from build123d import *

# Parameters (mm, degrees)
SALIENTE_EXTRUIR1_DEPTH = 30
CORTAR_EXTRUIR1_DEPTH   = 5
CROQUIS3_W              = 30.2
CROQUIS3_H              = 25.2
CORTAR_EXTRUIR2_DEPTH   = 2
CROQUIS4_R              = 1.1
CORTAR_EXTRUIR3_DEPTH   = 5
CROQUIS5_W              = 25.2
CROQUIS5_H              = 25.2
CORTAR_EXTRUIR4_DEPTH   = 2
REDONDEO2_R             = 8
REDONDEO3_R             = 2.7
CROQUIS6_W              = 8
CROQUIS6_H              = 14
SALIENTE_EXTRUIR2_DEPTH = 5
REDONDEO4_R             = 3
SALIENTE_EXTRUIR4_START = -2.4
SALIENTE_EXTRUIR4_DEPTH = 2.4
SALIENTE_EXTRUIR5_START = -30
SALIENTE_EXTRUIR5_DEPTH = 2.4
REDONDEO5_R             = 10
SALIENTE_EXTRUIR6_START = -5
SALIENTE_EXTRUIR6_DEPTH = 5
CORTAR_EXTRUIR6_START   = -2.4
CROQUIS14_R             = 1
CORTAR_EXTRUIR6_DEPTH   = 30
CROQUIS18_W             = 3
CROQUIS18_H             = 7.151114147
SALIENTE_EXTRUIR7_DEPTH = 5
CORTAR_EXTRUIR7_START   = -3
CORTAR_EXTRUIR7_DEPTH   = 3
CROQUIS22_R             = 1
CORTAR_EXTRUIR8_DEPTH   = 5
REDONDEO8_R             = 2
REDONDEO6_R             = 3


with BuildPart() as part:
    # Croquis1 → Saliente-Extruir1 (new body)
    with BuildSketch(Plane.XY):
        with BuildLine():
            Line((0, 0), (0, 5))
            Line((0, 5), (-40, 5))
            ThreePointArc((-40, 5), (-58.443639467, -0.437358826), (-71, -15))
            Line((-71, -15), (-71, -55))
            Line((-71, -55), (-66, -55))
            Line((-66, -55), (-66, -16.078431373))
            ThreePointArc((-66, -16.078431373), (-55.744135615, -4.621589797), (-41.078431373, 0))
            Line((-41.078431373, 0), (0, 0))
        make_face()
    extrude(amount=SALIENTE_EXTRUIR1_DEPTH)

    # Croquis2 → Cortar-Extruir1 (cut)
    with BuildSketch(Plane(origin=(0, 5, 0), x_dir=(1, 0, 0), z_dir=(0, 1, 0))):
        with BuildLine():
            Line((-18.4, -7.18), (-8.4, -7.18))
            ThreePointArc((-8.4, -7.18), (-7.3, -8.28), (-8.4, -9.38))
            Line((-8.4, -9.38), (-28.4, -9.38))
            ThreePointArc((-28.4, -9.38), (-29.5, -8.28), (-28.4, -7.18))
            Line((-28.4, -7.18), (-18.4, -7.18))
        make_face()
        with BuildLine():
            Line((-8.4, -20.62), (-28.4, -20.62))
            ThreePointArc((-28.4, -20.62), (-29.5, -21.72), (-28.4, -22.82))
            Line((-28.4, -22.82), (-18.4, -22.82))
            Line((-18.4, -22.82), (-8.4, -22.82))
            ThreePointArc((-8.4, -22.82), (-7.3, -21.72), (-8.4, -20.62))
        make_face()
    extrude(amount=-CORTAR_EXTRUIR1_DEPTH, mode=Mode.SUBTRACT)

    # Croquis3 → Cortar-Extruir2 (cut)
    with BuildSketch(Plane.XZ):
        with Locations((-18.4, 15)):
            Rectangle(CROQUIS3_W, CROQUIS3_H)
    extrude(amount=-CORTAR_EXTRUIR2_DEPTH, mode=Mode.SUBTRACT)

    # Croquis4 → Cortar-Extruir3 (cut)
    with BuildSketch(Plane.ZY.offset(71)):
        with Locations((22.071067812, -29.528932188)):
            Circle(CROQUIS4_R)
        with Locations((22.071067812, -43.671067812)):
            Circle(CROQUIS4_R)
        with Locations((7.928932188, -43.671067812)):
            Circle(CROQUIS4_R)
        with Locations((7.928932188, -29.528932188)):
            Circle(CROQUIS4_R)
    extrude(amount=-CORTAR_EXTRUIR3_DEPTH, mode=Mode.SUBTRACT)

    # Croquis5 → Cortar-Extruir4 (cut)
    with BuildSketch(Plane.ZY.offset(71)):
        with Locations((15, -36.6)):
            Rectangle(CROQUIS5_W, CROQUIS5_H)
    extrude(amount=-CORTAR_EXTRUIR4_DEPTH, mode=Mode.SUBTRACT)

    # Redondeo2
    redondeo2_edges = [part.edges().sort_by_distance(p)[0] for p in [
        (0, 2.5, 0),
        (-71, -15, 15),
        (-68.5, -55, 30),
        (0, 2.5, 30),
        (-68.5, -55, 0),
    ]]
    fillet(redondeo2_edges, radius=REDONDEO2_R)

    # Redondeo3
    redondeo3_edges = [part.edges().sort_by_distance(p)[0] for p in [
        (-70, -24, 27.6),
        (-70, -49.2, 27.6),
        (-70, -49.2, 2.4),
        (-70, -24, 2.4),
        (-3.3, 1, 27.6),
        (-3.3, 1, 2.4),
        (-33.5, 1, 2.4),
        (-33.5, 1, 27.6),
    ]]
    fillet(redondeo3_edges, radius=REDONDEO3_R)

    # Croquis6 → Saliente-Extruir2 (add)
    with BuildSketch(Plane.XZ):
        with Locations((4, 15)):
            Rectangle(CROQUIS6_W, CROQUIS6_H)
    extrude(amount=-SALIENTE_EXTRUIR2_DEPTH)

    # Redondeo4
    redondeo4_edges = [part.edges().sort_by_distance(p)[0] for p in [
        (8, 2.5, 8),
        (8, 2.5, 22),
    ]]
    fillet(redondeo4_edges, radius=REDONDEO4_R)

    # Croquis11 → Saliente-Extruir4 (add)
    with BuildSketch(Plane.XY.offset(30).offset(SALIENTE_EXTRUIR4_START)):
        with BuildLine():
            Line((-41.078431373, 0), (-14.078431373, 0))
            Line((-14.078431373, 0), (-66, -20))
            Line((-66, -20), (-66, -16.078431373))
            ThreePointArc((-66, -16.078431373), (-55.744135615, -4.621589797), (-41.078431373, 0))
        make_face()
    extrude(amount=SALIENTE_EXTRUIR4_DEPTH)

    # Croquis11<2> → Saliente-Extruir5 (add)
    with BuildSketch(Plane.XY.offset(30).offset(SALIENTE_EXTRUIR5_START)):
        with BuildLine():
            Line((-41.078431373, 0), (-14.078431373, 0))
            Line((-14.078431373, 0), (-66, -20))
            Line((-66, -20), (-66, -16.078431373))
            ThreePointArc((-66, -16.078431373), (-55.744135615, -4.621589797), (-41.078431373, 0))
        make_face()
    extrude(amount=SALIENTE_EXTRUIR5_DEPTH)

    # Redondeo5
    redondeo5_edges = [part.edges().sort_by_distance(p)[0] for p in [
        (-14.078431373, 0, 28.8),
        (-66, -20, 28.8),
        (-66, -20, 1.2),
        (-14.078431373, 0, 1.2),
    ]]
    fillet(redondeo5_edges, radius=REDONDEO5_R)

    # Croquis12 → Saliente-Extruir6 (add)
    with BuildSketch(Plane.ZY.offset(71).offset(SALIENTE_EXTRUIR6_START)):
        with BuildLine():
            Line((10.5, -55), (19.5, -55))
            Line((19.5, -55), (22, -55))
            Line((22, -55), (19.5, -55.5))
            ThreePointArc((19.5, -55.5), (17.5, -57.5), (19.5, -59.5))
            Line((19.5, -59.5), (19.5, -60))
            Line((19.5, -60), (10.5, -60))
            Line((10.5, -60), (10.5, -59.5))
            ThreePointArc((10.5, -59.5), (12.5, -57.5), (10.5, -55.5))
            Line((10.5, -55.5), (8, -55))
            Line((8, -55), (10.5, -55))
        make_face()
    extrude(amount=SALIENTE_EXTRUIR6_DEPTH)

    # Croquis14 → Cortar-Extruir6 (cut)
    with BuildSketch(Plane.XY.offset(2.4).offset(CORTAR_EXTRUIR6_START)):
        with Locations((-41.078431373, -1.005)):
            Circle(CROQUIS14_R)
    extrude(amount=CORTAR_EXTRUIR6_DEPTH, mode=Mode.SUBTRACT)

    # Croquis18 → Saliente-Extruir7 (add)
    with BuildSketch(Plane.ZY.offset(71)):
        with Locations((23.4, -20.424442926)):
            Rectangle(CROQUIS18_W, CROQUIS18_H)
    extrude(amount=SALIENTE_EXTRUIR7_DEPTH)

    # Croquis19 → Cortar-Extruir7 (cut)
    with BuildSketch(Plane.XY.offset(24.9).offset(CORTAR_EXTRUIR7_START)):
        with BuildLine():
            Line((-72.625, -22.049442927), (-72.625, -24))
            Line((-72.625, -24), (-71, -24))
            Line((-71, -24), (-71, -20.424442927))
            ThreePointArc((-71, -20.424442927), (-73.774048519, -19.275394407), (-72.625, -22.049442927))
        make_face()
    extrude(amount=CORTAR_EXTRUIR7_DEPTH, mode=Mode.SUBTRACT)

    # Croquis22 → Cortar-Extruir8 (cut)
    with BuildSketch(Plane.XZ):
        with Locations((2.5, 22)):
            Circle(CROQUIS22_R)
        with Locations((2.5, 8)):
            Circle(CROQUIS22_R)
    extrude(amount=-CORTAR_EXTRUIR8_DEPTH, mode=Mode.SUBTRACT)

    # Redondeo8
    redondeo8_edges = [part.edges().sort_by_distance(p)[0] for p in [
        (-76, -16.848885853, 23.4),
        (-76, -24, 23.4),
    ]]
    fillet(redondeo8_edges, radius=REDONDEO8_R)

    # Cortar-Barrer1: sweep along a path in Croquis23
    with BuildLine(Plane.XY.offset(2.4)) as cortar_barrer1_path:
        Line((-33.5, 0), (-41.078431373, 0))
        ThreePointArc((-41.078431373, 0), (-46.058616362, -0.620868951), (-50.857769, -2.089151876))
    # Croquis24 → Cortar-Barrer1 (sweep, cut)
    with BuildSketch(Plane(origin=(-33.5, 0, 0), x_dir=(0, 0, -1), z_dir=(1, 0, 0))):
        with BuildLine():
            Line((-7, 0), (-23, 0))
            ThreePointArc((-23, 0), (-15, 1), (-7, 0))
        make_face()
    sweep(path=cortar_barrer1_path.line, transition=Transition.RIGHT, mode=Mode.SUBTRACT)

    # Redondeo6
    # the kernel refuses this fillet: 3 mm, written as the material it adds along each edge
    with BuildSketch(Plane(origin=(0, 0, 8), x_dir=(-0.1270760613131033, 0, -0.9918929753966144), z_dir=(0, 1, 0))) as redondeo6_piece_1:
        with BuildLine():
            CenterArc((2.414445165, -2.975678926), REDONDEO6_R, 97.300661555, 52.967156255)
            Line((-0.190614092, -1.487839463), (-0.242715277, -1.458082674))
            ThreePointArc((-0.242715277, -1.458082674), (-0.154820625, -0.736295168), (-0.059513579, 0.007624564))
            Line((-0.059513579, 0.007624564), (0.007624564, 0.059513579))
            ThreePointArc((0.007624564, 0.059513579), (1.016608491, -0.004856197), (2.025592417, 0.059513579))
            Line((2.025592417, 0.059513579), (2.033216981, 0))
        make_face()
    extrude(amount=5)
    with BuildSketch(Plane(origin=(0, 0, 22), x_dir=(-0.12707606131310373, 0, 0.9918929753966141), z_dir=(0, 1, 0))) as redondeo6_piece_2:
        with BuildLine():
            CenterArc((2.414445165, 2.975678926), REDONDEO6_R, 209.73218219, 52.967156255)
            Line((-0.190614092, 1.487839463), (-0.242715277, 1.458082674))
            ThreePointArc((-0.242715277, 1.458082674), (-0.154820625, 0.736295168), (-0.059513579, -0.007624564))
            Line((-0.059513579, -0.007624564), (0.007624564, -0.059513579))
            ThreePointArc((0.007624564, -0.059513579), (1.016608491, 0.004856197), (2.025592417, -0.059513579))
            Line((2.025592417, -0.059513579), (2.033216981, 0))
        make_face()
    extrude(amount=5)


solid = part.part
The listing builds one solid part. Answer for the finished solid, in the listing's coordinates (mm). A direction names the side the tool comes from. Give positions to 0.01 mm unless a question says otherwise; leave off trailing zeros. Order: outer loops, then holes, each group sorted by start corner. A loop starts at its lowest first (then second) coordinate and runs counter-clockwise, first axis right, second up. Notation, with made-up numbers: (77.5, 66) - (125.5, 66) arc R24 cw to (125.5, 78) - close; hole circle Ø2 at (54.25, 66). An arc over 180 degrees is marked (long way). One line per item, written item: value. Start each with the question number.
1) Find the intervals of material crossed by L1, parallel to Z at x = -57, y = -8; L2, parallel to X at y = -17.5, z = 4.25; L3, parallel to Y at x = -5, z = 27.75, in increasing order.
2) A cutting plane is placed at A-A on y = -37. Give the vertices of the cut face in (x, z).
3) The mould has two halves that part along Y. Classify faces 1 (the face through (-70, -49.2, 15)), 2 (the face through (-29.5, 3.5, 8.3)), 3 (the face through (-67.521, -44.745, 7.69)), 4 (the face through (-75.4, -17.42, 23.42)): released by +Y, released by -Y, zero draft, split by the parting line, or undercut.
4) A cutting plane is placed at C-C on x = -64.5. Give the vertices of the cut face in (y, z), then the cut area to 3 significant figures.
5) A cutting plane is placed at B-B on x = -23. Give the vertices of the cut face in (y, z).
6) Given pin 1 Ø2 at (y, z) = (-25.5, 6) entering from +X; pin 2 Ø5 at (x, z) = (-21, 26.5) entering from -Y; pin 3 Ø4 at (x, y) = (-73.5, -20) entering from -Z, each flat-ended and moving along its own axis, determine where each tip first touches the part or whether it passes through.
7) A tool of negligible diameter and unlimited length cuts with its end or side. For faces 5 (the face through (-7.3, 3.5, 8.3)), 6 (the face through (-32.73, 1.01, 3.21)), 7 (the face through (-70, -37, 27.6)), from which of +Z, -Z, +X, -X, +Y, -Y can it reach the whole face along a straight path? Write none if from no direction.
8) A cutting plane is placed at D-D on y = -57.5. Give the vertices of the cut face in (x, z), then the cut area to 3 significant figures.
Answer sheet:
1. L1: z = 0 to 2.4, 27.6 to 30
1. L2: x = -71 to -66
1. L3: y = 0 to 5
2. outline: (-71, 0) - (-66, 0) - (-66, 30) - (-71, 30) - (-71, 27.6) - (-69, 27.6) - (-69, 2.4) - (-71, 2.4) - close
3. face 1: undercut
3. face 2: zero draft
3. face 3: undercut
3. face 4: released by +Y
4. outline: (-21.6, 0) - (-5.42, 0) - (-5.42, 30) - (-21.6, 30) - (-21.6, 27.6) - (-13.43, 27.6) - (-13.43, 2.4) - (-21.6, 2.4) - close
4. area: 279 mm2
5. outline: (-3.44, 0) - (5, 0) - (5, 7.18) - (2, 7.18) - (2, 2.4) - (-3.44, 2.4) - close; (-3.44, 27.6) - (2, 27.6) - (2, 22.82) - (5, 22.82) - (5, 30) - (-3.44, 30) - close; (2, 9.38) - (5, 9.38) - (5, 20.62) - (2, 20.62) - close
6. pin 1: stops at x = -66
6. pin 2: stops at y = -3.53
6. pin 3: stops at z = 21.9
7. face 5: +Y, -Y
7. face 6: -Y
7. face 7: -X
8. outline: (-71, 12.5) - (-66, 12.5) - (-66, 17.5) - (-71, 17.5) - close
8. area: 25.0 mm2
